Geometry: final body of the model. Coordinates: model frame, mm. Face numbers are marked on the shaded views. Round coordinates to 2 decimals unless told otherwise and drop trailing zeros. Loops run counter-clockwise (first coordinate to the right, second up) from the corner with the lowest first, then second, coordinate; pieces in that order, holes last. Notation, with made-up numbers: M -33,50.5 L 23,50.5 A24 cw 23,80.5 Z; hole C 86.5,63.5 d9. An arc over 180 degrees is marked long. Return JSON: item names as keys, results as strings.
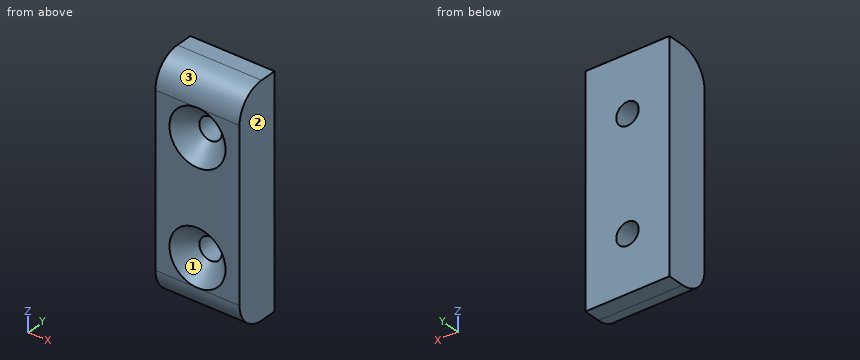
from build123d import *

# Parameters (mm, degrees)
F0_R     = 2
F1_DEPTH = 8
F2_SIZE  = 3
F3_R     = 4.99999


# Not quite as in the source:
# - a fillet or chamfer is up to 0.001 mm smaller than in the source, because OpenCascade refuses the exact size


with BuildPart() as f1:
    # F0 (on Front) → F1 (new body)
    with BuildSketch(Plane.XZ):
        Polygon((0, 20), (0, 0), (0, -20), (15, -20), (15, 0), (15, 20), align=None)
        with Locations((7.5, -10)):
            Circle(F0_R, mode=Mode.SUBTRACT)
        with Locations((7.5, 10)):
            Circle(F0_R, mode=Mode.SUBTRACT)
    extrude(amount=F1_DEPTH)

    # F2
    f2_edges = [f1.edges().sort_by_distance(p)[0] for p in [
        (5.5, -8, 10),
        (5.5, -8, -10),
    ]]
    chamfer(f2_edges, length=F2_SIZE)

    # F3 (radius 5 in the source; OpenCascade refuses exactly that, so slightly less here)
    f3_edges = [f1.edges().sort_by_distance(p)[0] for p in [
        (7.5, -8, 20),
        (7.5, -8, -20),
    ]]
    fillet(f3_edges, radius=F3_R)


solid = f1.part
Q1. Material intervals for L1, parallel to Z at x = 7.5, y = -3.2; L2, parallel to Z at x = 7, y = -0.5; L3, parallel to Z at x = 1.75, y = -3.25, sorted ascending.
Determined:
{"L1": "z = -20 to -12, -8 to 8, 12 to 20", "L2": "z = -20 to -11.94, -8.06 to 8.06, 11.94 to 20", "L3": "z = -19.99 to 19.99"}
Q2. Pin query (flat end, axial travel): pin 1 (2 mm diameter, centred on x = 8, z = 11.5, fed in from -Y); pin 2 (2 mm diameter, centred on x = 5.5, y = -6, fed in from +Z). Return the tip coordinate at first contact, or that it passes through.
Determined:
{"pin 1": "stops at y = -5.58", "pin 2": "stops at z = 19.58"}
Q3. Section query B-B (z = 10). Output: boundary loops of the cut face in (x, y).
Determined:
{"outline": "M 0,-8 L 2.5,-8 L 5.5,-5 L 5.5,0 L 0,0 Z; M 9.5,-5 L 12.5,-8 L 15,-8 L 15,0 L 9.5,0 Z"}
Q4. Section query C-C (y = -7). Output: boundary loops of the cut face in (x, z), plus the area to 3 significant figures.
Determined:
{"outline": "M 0,-18 L 15,-18 L 15,18 L 0,18 Z; hole C 7.5,-10 d8; hole C 7.5,10 d8", "area": "439 mm^2"}
Q5. Section query D-D (y = -1.75). Output: boundary loops of the cut face in (x, z), plus the area to 3 significant figures.
Determined:
{"outline": "M 0,-20 L 15,-20 L 15,20 L 0,20 Z; hole C 7.5,-10 d4; hole C 7.5,10 d4", "area": "575 mm^2"}
Q6. Section query A-A (x = 7.5). State how many separate pieces and enclosed holes the cut face has, plus the area to 3 significant figures.
Determined:
{"separate pieces": "3", "enclosed holes": "0", "area": "227 mm^2"}
Q7. Pull-direction query (X, two-part tool) for the marked faces 1, 2 and 3; classes: pulls with the +X half, pulls with the -X half, needs draft (parallel to the pull), parting line crosses it, or undercut.
Determined:
{"face 1": "undercut", "face 2": "pulls with the +X half", "face 3": "needs draft"}
